Geometry check sheet. Reference: the model listing, model coordinates, mm. A direction names the side the tool comes from. Round coordinates to 2 decimals unless told otherwise and drop trailing zeros. Write each loop counter-clockwise with the first axis right and the second up, starting at its lowest first coordinate (ties: lowest second). Pieces come first, ordered by that corner, then holes. Notation, with made-up numbers: M -33.5,48 L 23.5,48 A29 cw 23.5,87 Z; hole C -11,57.5 d2. An arc over 180 degrees is marked long. Use a Markdown table: item, result.
Autodesk Inventor part; units mm, degrees
ref_plane "YZ Plane" through (0, 0, 0) normal (1, 0, 0) x (0, 1, 0)
ref_plane "XZ Plane" through (0, 0, 0) normal (0, 1, 0) x (-1, 0, 0)
ref_plane "XY Plane" through (0, 0, 0) normal (0, 0, 1) x (1, 0, 0)
sketch "Arduino Uno" plane through (0, 0, 0) normal (0, 0, 1) x (1, 0, 0)
  line L0 (0, 0) -> (68.6, 0)
  line L1 (68.6, 0) -> (68.6, 53.3)
  line L2 (68.6, 53.3) -> (0, 53.3)
  line L3 (0, 53.3) -> (0, 0)
  circle A0 centre (14, 2.5) radius 1.5
  circle A1 centre (66.1, 5.1) radius 1.5
  circle A2 centre (66.1, 33) radius 1.5
  circle A3 centre (15.3, 48.2) radius 1.5
  dimension "d6" = 68.6
  dimension "d7" = 53.3
  dimension "d97" = 3
  dimension "d98" = 14
  dimension "d99" = 2.5
  dimension "d100" = 3
  dimension "d101" = 5.1
  dimension "d102" = 66.1
  dimension "d103" = 33
  dimension "d105" = 66.1
  dimension "d106" = 3
  dimension "d107" = 3
  dimension "d108" = 48.2
  dimension "d109" = 15.3
sketch "Sketch2" plane through (0, 0, 0) normal (0, 0, 1) x (1, 0, 0)
  line L0 (-7.6136, -10.2044) -> (-7.6136, 63.0956)
  line L1 (-7.6136, 63.0956) -> (106.3864, 63.0956)
  line L2 (106.3864, 63.0956) -> (106.3864, -10.2044)
  line L3 (106.3864, -10.2044) -> (-7.6136, -10.2044)
  dimension "d29" = 114
  dimension "d39" = 73.3
extrude "Back Plate" add sketch "Sketch2" against normal blind 10
extrude "Uno Mounting Holes" cut sketch "Arduino Uno" against normal blind 5 contours A0 | A1 | A2 | A3
sketch "3.5\" TFT LCD Screen" plane through (0, 0, 0) normal (0, 0, 1) x (1, 0, 0)
  line L0 (88.6005, 0.0003) -> (88.6005, 53.3003)
  line L1 (88.6005, 53.3003) -> (10.6005, 53.3003)
  line L2 (10.6005, 53.3003) -> (10.6005, 0.0003)
  line L3 (10.6005, 0.0003) -> (88.6005, 0.0003)
  line L4 (-7.6136, -10.2044) -> (-7.6136, 63.0956)
  line L5 (106.3864, -10.2044) -> (-7.6136, -10.2044)
  line L6 (106.3864, 63.0956) -> (106.3864, -10.2044)
  line L7 (-7.6136, 63.0956) -> (106.3864, 63.0956)
  point P0 (0, 0)
  point P1 (68.6, 0)
  dimension "d35" = 78
  dimension "d36" = 53.3
  dimension "d37" = 78
  dimension "d38" = 53.3
sketch "SD Card Slot" plane through (0, 0, 0) normal (0, 0, 1) x (1, 0, 0)
  line L0 (43.3864, 9.1) -> (-7.6136, 9.1)
  line L1 (-7.6136, 9.1) -> (-7.6136, 44.1)
  line L2 (-7.6136, 44.1) -> (43.3864, 44.1)
  line L3 (43.3864, 44.1) -> (43.3864, 9.1)
  circle A0 centre (14, 2.5) radius 1.6
  line L4 (-7.6136, -10.2044) -> (-7.6136, 63.0956)
  circle A1 centre (15.3, 50.7) radius 1.6
  point P0 (0, 0)
  dimension "d41" = 35
  dimension "d42" = 51
  dimension "d44" = 6.6
  dimension "d45" = 0
sketch "Sketch5" plane through (0, 0, 0) normal (0, 0, 1) x (1, 0, 0)
  line L0 (43.3864, 9.1) -> (-7.6136, 9.1)
  line L1 (43.3864, 44.1) -> (43.3864, 9.1)
  line L2 (-7.6136, 44.1) -> (43.3864, 44.1)
  line L3 (-7.6136, 9.1) -> (-7.6136, 44.1)
  line L4 (40.3864, 7.5) -> (40.3864, 43.5)
  line L5 (40.3864, 7.5) -> (-7.6136, 7.5)
  line L6 (-7.6136, -10.2044) -> (-7.6136, 63.0956)
  line L7 (40.3864, 43.5) -> (-7.6136, 43.5)
  line L8 (-7.6136, 43.5) -> (-7.6136, 46)
  line L9 (-7.6136, 46) -> (44.3864, 46)
  line L10 (-7.6136, 7.5) -> (-7.6136, 5)
  line L11 (-7.6136, 5) -> (44.3864, 5)
  line L12 (44.3864, 5) -> (44.3864, 46)
  circle A0 centre (15.3, 48.2) radius 1.5
  circle A1 centre (14, 2.5) radius 1.5
  point P0 (0, 0)
  dimension "d47" = 2.5
  dimension "d48" = 52
  dimension "d49" = 2.5
  dimension "d115" = 41
  dimension "d116" = 36
  dimension "d117" = 1
extrude "SD Card Slot Slot" add sketch "Sketch5" along normal blind 10 contours L1 L2 L6 L9 L12 L11 L5 L4 L0 | L0 L4 L7 L3 L2 L1
sketch "Sketch6" plane through (44.3864, 5, 0) normal (1, 0, 0) x (0, 0, -1)
  line L0 (0, 41) -> (0, 0)
  line L1 (0, 41) -> (-10, 41)
  line L2 (-10, 0) -> (-10, 41)
  line L3 (0, 0) -> (-10, 0)
  line L4 (-6, 37) -> (-4, 37)
  line L5 (-4, 37) -> (-4, 4)
  line L6 (-4, 4) -> (-6, 4)
  line L7 (-6, 4) -> (-6, 37)
  point P0 (0, -5)
  dimension "d52" = 4
extrude "SD Ribbon Slot" cut sketch "Sketch6" against normal through all contours L4 L5 L6 L7
fillet "1.2mm Fillet" [suppressed]
sketch "Sketch7" plane through (0, 0, 0) normal (0, 0, 1) x (1, 0, 0)
  line L0 (106.3864, -10.2044) -> (101.3864, -10.2044)
  line L1 (101.3864, -10.2044) -> (101.3864, -5.2044)
  line L2 (101.3864, -5.2044) -> (106.3864, -5.2044)
  line L3 (106.3864, -5.2044) -> (106.3864, -10.2044)
  line L4 (49.3864, -10.2044) -> (49.3864, 80.0118)
  line L5 (-7.6136, 63.0956) -> (106.3864, 63.0956)
  line L6 (106.3864, 26.4456) -> (-34.6963, 26.4456)
  line L7 (-7.6136, -10.2044) -> (-2.6136, -10.2044)
  line L8 (-2.6136, -10.2044) -> (-2.6136, -5.2044)
  line L9 (-2.6136, -5.2044) -> (-7.6136, -5.2044)
  line L10 (-7.6136, -5.2044) -> (-7.6136, -10.2044)
  line L11 (106.3864, 63.0956) -> (101.3864, 63.0956)
  line L12 (101.3864, 63.0956) -> (101.3864, 58.0956)
  line L13 (101.3864, 58.0956) -> (106.3864, 58.0956)
  line L14 (106.3864, 58.0956) -> (106.3864, 63.0956)
  line L15 (-7.6136, 63.0956) -> (-2.6136, 63.0956)
  line L16 (-2.6136, 63.0956) -> (-2.6136, 58.0956)
  line L17 (-2.6136, 58.0956) -> (-7.6136, 58.0956)
  line L18 (-7.6136, 58.0956) -> (-7.6136, 63.0956)
  point P0 (0, 0)
  point P1 (0, 52.8913)
  dimension "d56" = 5
  dimension "d57" = 5
  dimension "d58" = 57
  dimension "d59" = 36.65
extrude "Pillars" [suppressed]
sketch "Sketch8" plane through (0, 0, 31) normal (0, 0, 1) x (1, 0, 0)
  line L0 (101.3864, -10.2044) -> (-2.6136, -10.2044)
  line L1 (-7.6136, -5.2044) -> (-2.6136, -5.2044)
  line L2 (101.3864, -10.2044) -> (-2.6136, -10.2044)
  line L3 (-2.6136, -10.2044) -> (-2.6136, -5.2044)
  line L4 (-2.6136, -5.2044) -> (101.3864, -5.2044)
  line L5 (101.3864, -5.2044) -> (101.3864, -10.2044)
  line L6 (101.3864, 63.0956) -> (101.3864, 58.0956)
  line L7 (106.3864, 63.0956) -> (106.3864, -10.2044)
  line L8 (101.3864, 58.0956) -> (106.3864, 58.0956)
  line L9 (106.3864, 58.0956) -> (106.3864, -5.2044)
  line L10 (106.3864, -5.2044) -> (101.3864, -5.2044)
  line L11 (101.3864, -5.2044) -> (101.3864, 58.0956)
  line L12 (-7.6136, 58.0956) -> (-2.6136, 58.0956)
  line L13 (-7.6136, 63.0956) -> (106.3864, 63.0956)
  line L14 (-2.6136, 58.0956) -> (101.3864, 58.0956)
  line L15 (101.3864, 58.0956) -> (101.3864, 63.0956)
  line L16 (101.3864, 63.0956) -> (-2.6136, 63.0956)
  line L17 (-2.6136, 63.0956) -> (-2.6136, 58.0956)
  line L18 (-2.6136, 58.0956) -> (-7.6136, 58.0956)
  line L19 (-7.6136, 58.0956) -> (-7.6136, -5.2044)
  line L20 (-7.6136, -5.2044) -> (-2.6136, -5.2044)
  line L21 (-2.6136, -5.2044) -> (-2.6136, 58.0956)
  point P0 (0, 0)
extrude "Beams (Will they print?)" [suppressed]
sketch "Sketch9" plane through (0, 0, 0) normal (0, 0, 1) x (1, 0, 0)
  line L0 (106.3864, 63.0956) -> (106.3864, -10.2044)
  line L1 (-7.6136, -10.2044) -> (-7.6136, 63.0956)
  line L2 (106.3864, -10.2044) -> (-7.6136, -10.2044)
  line L3 (-7.6136, -10.2044) -> (-7.6136, 63.0956)
  line L4 (-7.6136, 63.0956) -> (106.3864, 63.0956)
  line L5 (-7.6136, 63.0956) -> (106.3864, 63.0956)
  line L6 (106.3864, 63.0956) -> (106.3864, -10.2044)
  line L7 (106.3864, -10.2044) -> (106.3864, -15.2044)
  line L8 (106.3864, -15.2044) -> (-7.6136, -15.2044)
  line L9 (-7.6136, -15.2044) -> (-12.6136, -15.2044)
  line L10 (-12.6136, -15.2044) -> (-12.6136, 63.0956)
  line L11 (-12.6136, 63.0956) -> (-12.6136, 68.0956)
  line L12 (-12.6136, 68.0956) -> (106.3864, 68.0956)
  line L13 (106.3864, 68.0956) -> (111.3864, 68.0956)
  line L14 (111.3864, 68.0956) -> (111.3864, -15.2044)
  line L15 (111.3864, -15.2044) -> (106.3864, -15.2044)
  point P0 (0, 0)
  dimension "d64" = 5
  dimension "d65" = 5
  dimension "d66" = 5
  dimension "d67" = 5
extrude "Outer Walls (5mm Offset)" add sketch "Sketch9" along normal blind 31 and the other way blind 10
extrude "Extrusion9" [suppressed]
sketch "Sketch10" plane through (-12.6136, -15.2044, 31) normal (-1, 0, 0) x (0, 0, 1)
  line L0 (-31, 63.5044) -> (-31, 78.3)
  line L1 (-13.6, 56.6044) -> (-2.9, 56.6044)
  line L2 (-2.9, 56.6044) -> (-2.9, 44.6044)
  line L3 (-2.9, 44.6044) -> (-13.6, 44.6044)
  line L4 (-13.6, 44.6044) -> (-13.6, 56.6044)
  line L5 (-1.9, 43.6044) -> (-1.9, 57.6044)
  line L6 (-1.9, 57.6044) -> (-14.6, 57.6044)
  line L7 (-14.6, 57.6044) -> (-14.6, 43.6044)
  line L8 (-14.6, 43.6044) -> (-1.9, 43.6044)
  line L9 (-25, 57.2044) -> (-25, 24.2044)
  line L10 (-25, 24.2044) -> (-27, 24.2044)
  line L11 (-27, 24.2044) -> (-27, 57.2044)
  line L12 (-27, 57.2044) -> (-25, 57.2044)
  line L13 (-31, 22.7044) -> (-31, 58.7044)
  line L14 (-31, 22.7044) -> (-21, 22.7044)
  line L15 (-21, 58.7044) -> (-21, 22.7044)
  line L16 (-31, 58.7044) -> (-21, 58.7044)
  point P0 (-31, 68.5047)
  dimension "d82" = 10.7
  dimension "d83" = 12
  dimension "d84" = 1
extrude "SD Card Opening" cut sketch "Sketch10" against normal blind 5 contours L1 L2 L3 L4 | L8 L7 L6 L5 | L9 L10 L11 L12 | L13 L16 L15 L14
fillet "4mm Fillet" radius 4 8 edges at (-12.6136, 68.0956, 10.5) (-12.6136, -15.2044, 10.5) (111.3864, -15.2044, 10.5) (111.3864, 68.0956, 10.5) (49.3864, 68.0956, -10) (-12.6136, 26.4456, -10) (49.3864, -15.2044, -10) (111.3864, 26.4456, -10)
sketch "Sketch11" plane through (0, 0, 0) normal (0, 0, 1) x (1, 0, 0)
  line L0 (98.4778, 47.4456) -> (98.4778, 5.4456) construction
  line L1 (98.4778, 5.4456) -> (86.054, 5.4456) construction
  line L2 (86.054, 5.4456) -> (86.054, 47.4456) construction
  line L3 (86.054, 47.4456) -> (98.4778, 47.4456) construction
  line L4 (-8.6136, 68.0956) -> (107.3864, 68.0956)
  line L5 (107.3864, 68.0956) -> (107.3864, 26.4456)
  line L6 (107.3864, 26.4456) -> (48.9636, 26.4456)
  point P0 (0, 0)
  dimension "d88" = 41.65
  dimension "d89" = 42
  dimension "d90" = 21
feature "Inside Text" [suppressed]
sketch "Sketch12" plane through (0, 0, 31) normal (0, 0, 1) x (1, 0, 0)
  circle A0 centre (108.3864, -12.2044) radius 1.5
  line L0 (-12.6136, -15.2044) -> (111.3864, -15.2044)
  line L1 (111.3864, -15.2044) -> (111.3864, 68.0956)
  line L2 (107.3864, -15.2044) -> (-8.6136, -15.2044)
  line L3 (49.3864, -15.2044) -> (49.3864, 77.1219)
  line L4 (-8.6136, -11.2044) -> (-12.6136, -11.2044)
  line L5 (-12.6136, -11.2044) -> (-12.6136, 26.4456)
  line L6 (-12.6136, -11.2044) -> (-12.6136, 64.0956)
  line L7 (-12.6136, 26.4456) -> (133.0429, 26.4456)
  circle A1 centre (-9.6136, -12.2044) radius 1.5
  line L8 (111.3864, 26.4456) -> (-34.2702, 26.4456)
  circle A2 centre (108.3864, 65.0956) radius 1.5
  line L9 (-8.6136, 64.0956) -> (-12.6136, 64.0956)
  circle A3 centre (-9.6136, 65.0956) radius 1.5
  point P0 (0, 0)
  point P1 (111.3864, -11.2044)
  point P2 (111.3864, 64.0956)
  dimension "d91" = 3
  dimension "d92" = 3
  dimension "d93" = 3
  dimension "d94" = 37.65
extrude "3mm Screw Holes" cut sketch "Sketch12" against normal blind 15 contours A0 | A1 | A2 | A3
sketch "Sketch15" plane through (-12.6136, -11.2044, 31) normal (-1, 0, 0) x (0, 0, 1)
  line L0 (-31, 54.7044) -> (-21, 54.7044)
  line L1 (-21, 54.7044) -> (-31, 54.7044)
  line L2 (-31, 54.7044) -> (-31, 53.6284)
  line L3 (-31, 53.6284) -> (-21, 53.6284)
  line L4 (-21, 53.6284) -> (-21, 54.7044)
  line L5 (-21, 36.7044) -> (-31, 36.7044)
  line L6 (-31, 18.7044) -> (-21, 18.7044)
  line L7 (-21, 18.7044) -> (-31, 18.7044)
  line L8 (-31, 18.7044) -> (-31, 19.7803)
  line L9 (-31, 19.7803) -> (-21, 19.7803)
  line L10 (-21, 19.7803) -> (-21, 18.7044)
  point P0 (-31, 11.2044)
  dimension "d123" = 18
extrude "Extra Walls" add sketch "Sketch15" against normal blind 2
properties part number "Back Plate test05"
Item 1: Cross-section at A-A, the plane y = 33. Record the cut outline in (x, z), and give its area (3 significant figures).
Outcome:
| item | result |
|---|---|
| outline | M -12.61,-6 A4 ccw -8.61,-10 L 107.39,-10 A4 ccw 111.39,-6 L 111.39,31 L 106.39,31 L 106.39,0 L 67.6,0 L 67.6,-5 L 64.6,-5 L 64.6,0 L 44.39,0 L 44.39,4 L 40.39,4 L 40.39,0 L -12.61,0 Z; M -12.61,10 L -7.61,10 L -7.61,16.4 L -12.61,16.4 Z; M -12.61,29.1 L -7.61,29.1 L -7.61,31 L -12.61,31 Z; M 40.39,6 L 44.39,6 L 44.39,10 L 40.39,10 Z |
| area | 1,450 mm2 |
Item 2: Material ranges on line 1 along Y through (x, z) = (12.5, 1); line 2 along Y through (x, z) = (81.5, 9); line 3 along X through (y, z) = (-2, 10), recorded low to high. Write a range as from..to.
Outcome:
| item | result |
|---|---|
| line 1 | y = -15.2..-10.2, 5..7.5, 43.5..46, 63.1..68.1 |
| line 2 | y = -15.2..-10.2, 63.1..68.1 |
| line 3 | x = -12.61..-7.61, 106.39..111.39 |
Item 3: Mould release check, pull along Z, two halves, no side actions. Record for faces 1 (the face through (-10, -12, 16)), 2 (the face through (-9.809, 66.583, 23.605)), 3 (the face through (-10, 42.4, 23)): +Z half, -Z half, draft (parallel to the pull), parting line (faces both ways), or undercut.
Outcome:
| item | result |
|---|---|
| face 1 | +Z half |
| face 2 | draft |
| face 3 | undercut |
Item 4: Cross-section at C-C, the plane y = 52.5. Record the cut outline in (x, z), and give its area (3 significant figures).
Outcome:
| item | result |
|---|---|
| outline | M -12.61,-6 A4 ccw -8.61,-10 L 107.39,-10 A4 ccw 111.39,-6 L 111.39,31 L 106.39,31 L 106.39,0 L -7.61,0 L -7.61,31 L -12.61,31 Z |
| area | 1,540 mm2 |
Item 5: Cross-section at B-B, the plane x = 71. Record the cut outline in (y, z), and give its area (3 significant figures).
Outcome:
| item | result |
|---|---|
| outline | M -15.2,-6 A4 ccw -11.2,-10 L 64.1,-10 A4 ccw 68.1,-6 L 68.1,31 L 63.1,31 L 63.1,0 L -10.2,0 L -10.2,31 L -15.2,31 Z |
| area | 1,140 mm2 |
Item 6: Cross-section at D-D, the plane x = 33.5. Record the cut outline in (y, z).
Outcome:
| item | result |
|---|---|
| outline | M -15.2,-6 A4 ccw -11.2,-10 L 64.1,-10 A4 ccw 68.1,-6 L 68.1,31 L 63.1,31 L 63.1,0 L 46,0 L 46,10 L 43.5,10 L 43.5,0 L 7.5,0 L 7.5,10 L 5,10 L 5,0 L -10.2,0 L -10.2,31 L -15.2,31 Z |
Item 7: Access from +Z, -Z, +X, -X, +Y, -Y to the whole of each face (thin tool, end or side, straight path). Record for faces 4 (the face through (-10, 28.4, 23)), 5 (the face through (111.386, 27, 12)), 6 (the face through (16.73, 48.65, -2.46)).
Outcome:
| item | result |
|---|---|
| face 4 | -X |
| face 5 | +Z, -Z, +X, +Y, -Y |
| face 6 | +Z |
Item 8: Go/stop test with flat-tipped pins: pin 1 (4 mm diameter, centred on x = -9.61, y = -12.2, fed in from -Z); pin 2 (8 mm diameter, centred on x = 65, y = 49.5, fed in from +Z); pin 3 (4.5 mm diameter, centred on x = 43, y = 24, fed in from +Z); pin 4 (1 mm diameter, centred on x = -11.5, z = 4, fed in from +Y). Record where each tip stops, or that it passes through.
Outcome:
| item | result |
|---|---|
| pin 1 | stops at z = -10 |
| pin 2 | stops at z = 0 |
| pin 3 | stops at z = 10 |
| pin 4 | stops at y = 67.31 |
